Geometry: see drawing. Coordinates: mm, zero at the bounding-box minimum. Coordinates: 2 decimals unless noted, no trailing zeros. Order: outer loops, then holes, each group sorted by start corner. A loop starts at its lowest first (then second) coordinate and runs counter-clockwise, first axis right, second up.
Item 1: Ray query, line 1 (Y direction, x = 13, z = 6); line 2 (Y direction, x = 14, z = 5.5); line 3 (X direction, y = 269.5, z = 1.5). Return the intervals inside material, ascending.
Item 2: Section D-D on x = 7.62. Return the cut outline in (y, z).
Item 3: Contact query for flat-ended pins moving along their axis: P1, Ø3, axis at x = 8, z = 3.5, coming from the +Y side; P2, Ø1.9, axis at y = 101, z = 4, coming from the +X side (3 decimals); P3, Ø1.5, axis at x = 143.5, z = 0.5, coming from the +Y side. Output: stop coordinate, or through.
Item 4: Section C-C on x = 165. State how many separate pieces and enclosed holes the cut face has, then the cut area to 3 significant figures.
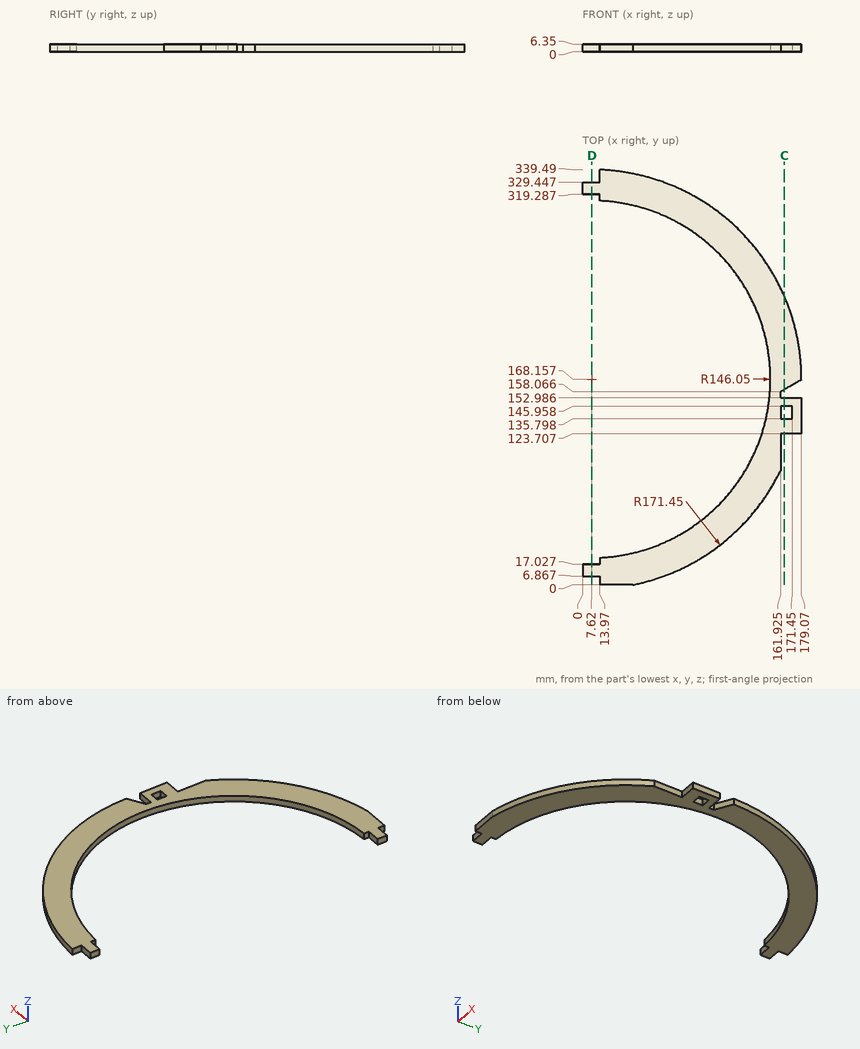
Answer list:
1. line 1: y = 6.87 to 17.03, 319.29 to 329.45
1. line 2: y = 0 to 22.25, 314.07 to 339.49
1. line 3: x = 112.79 to 145.91
2. outline: (6.87, 0) - (17.03, 0) - (17.03, 6.35) - (6.87, 6.35) - close; (319.29, 0) - (329.45, 0) - (329.45, 6.35) - (319.29, 6.35) - close
3. P1: stops at y = 329.45
3. P2: stops at x = 161.925
3. P3: stops at y = 273.68
4. separate pieces: 3
4. enclosed holes: 0
4. area: 606 mm2
